Autodesk Inventor part; units mm, degrees
ref_plane "YZ Plane" through (0, 0, 0) normal (1, 0, 0) x (0, 1, 0)
ref_plane "XZ Plane" through (0, 0, 0) normal (0, 1, 0) x (-1, 0, 0)
ref_plane "XY Plane" through (0, 0, 0) normal (0, 0, 1) x (1, 0, 0)
sketch "Sketch1" plane through (0, 0, 0) normal (0, 0, 1) x (1, 0, 0)
  line L0 (0, 0) -> (300, 0)
  line L1 (300, 0) -> (300, 200)
  line L2 (300, 200) -> (0, 200)
  line L3 (0, 200) -> (0, 0)
  dimension "d0" = 300
  dimension "d1" = 200
extrude "Extrusion1" add sketch "Sketch1" along normal blind 12
sketch "Sketch2" plane through (0, 0, 0) normal (0, 0, -1) x (-1, 0, 0)
  line L0 (-250, 150) -> (-50, 150)
  line L1 (-50, 150) -> (-50, 50)
  line L2 (-50, 50) -> (-250, 50)
  line L3 (-250, 50) -> (-250, 150)
  point P0 (0, 0)
  dimension "d4" = 200
  dimension "d5" = 100
extrude "Extrusion2" cut sketch "Sketch2" against normal blind 19
sketch "Sketch3" plane through (0, 0, 12) normal (0, 0, 1) x (1, 0, 0)
  line L0 (0, 0) -> (300, 0)
  line L1 (300, 0) -> (250, 0)
  line L2 (250, 0) -> (250, 200)
  line L3 (250, 200) -> (300, 200)
  line L4 (300, 200) -> (300, 0)
  line L5 (0, 0) -> (50, 0)
  line L6 (50, 0) -> (50, 200)
  line L7 (50, 200) -> (0, 200)
  line L8 (0, 200) -> (0, 0)
  dimension "d8" = 50
  dimension "d9" = 200
  dimension "d10" = 50
  dimension "d11" = 200
extrude "Extrusion3" add sketch "Sketch3" along normal blind 50
sketch "Sketch4" plane through (0, 0, 0) normal (-1, 0, 0) x (0, 0, 1)
  point P0 (0, 0)
sketch "Sketch5" plane through (0, 0, 0) normal (-1, 0, 0) x (0, 0, 1)
  circle A0 centre (37, 35) radius 4
  circle A1 centre (37, 100) radius 6.5
  circle A2 centre (37, 165) radius 4
  point P0 (0, 0)
  dimension "d14" = 8
  dimension "d15" = 13
  dimension "d16" = 8
extrude "Extrusion4" cut sketch "Sketch5" against normal blind 900
chamfer "Chamfer1" distance 5 angle 45 9 edges at (0, 100, 62) (0, 0, 31) (25, 0, 62) (275, 0, 62) (300, 100, 62) (275, 200, 62) (300, 200, 31) (0, 200, 31) (300, 0, 31)
properties part number "base box"
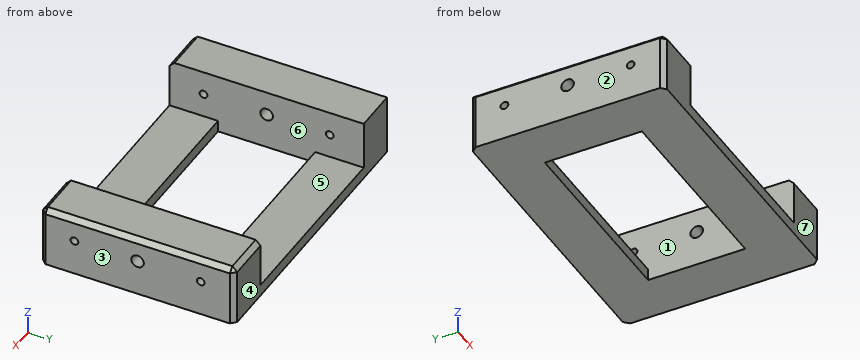
Source: CAD feature listing. Evaluate the final solid. Frame: model axes, mm. Face numbers are marked on the shaded views. A direction names the side the tool comes from. Give positions to 0.01 mm unless a question says otherwise; leave off trailing zeros. Loops run counter-clockwise (first coordinate to the right, second up) from the corner with the lowest first, then second, coordinate; pieces in that order, holes last. Notation, with made-up numbers: (-1, 49) -> (14, 49) arc R16 ccw to (14, 54) -> close; hole circle Ø7 at (-5.5, -1.5). An arc over 180 degrees is marked (long way). Use a Markdown table: item, result. Add a question column.
(1) Ray query, line 1 (Y direction, x = 11, z = 37); line 2 (X direction, y = 96, z = 4); line 3 (Y direction, x = 42, z = 38). Return the intervals inside material, ascending.
(2) First-contact query: pin 1 Ø8 at (x, y) = (200.5, 156.5) entering from +Z. Flat tip, straight axial feed; report the tip coordinate or a pass-through.
(3) Section query D-D (x = 91.5). Output: boundary loops of the cut face in (y, z), then the cut area to 3 significant figures.
(4) Section query A-A (y = 82). Output: boundary loops of the cut face in (x, z).
(5) Pull-direction query (X, two-part tool) for the marked faces 1, 2, 3 and 4; classes: +X half, -X half, draft (parallel to the pull), parting line (faces both ways), or undercut.
(6) Section query C-C (y = 165). Output: boundary loops of the cut face in (x, z).
(7) Access query for the marked faces 5, 6 and 7. Directions: +Z, -Z, +X, -X, +Y, -Y. A direction counts if a zero-diameter tool reaches every point of the face in a straight line with its end or side. Return the directions, or none.
(8) Section query B-B (z = 26). Output: boundary loops of the cut face in (x, y).
Checked values:
| question | item | result |
|---|---|---|
| 1 | line 1 | 0 to 31, 39 to 93.5, 106.5 to 161, 169 to 200 |
| 1 | line 2 | 0 to 50, 250 to 300 |
| 1 | line 3 | 0 to 31.13, 38.87 to 93.58, 106.42 to 161.13, 168.87 to 200 |
| 2 | pin 1 | z = 12 |
| 3 | outline | (0, 0) -> (50, 0) -> (50, 12) -> (0, 12) -> close; (150, 0) -> (200, 0) -> (200, 12) -> (150, 12) -> close |
| 3 | area | 1,200 mm^2 |
| 4 | outline | (0, 0) -> (50, 0) -> (50, 62) -> (5, 62) -> (0, 57) -> close; (250, 0) -> (300, 0) -> (300, 57) -> (295, 62) -> (250, 62) -> close |
| 5 | face 1 | undercut |
| 5 | face 2 | -X half |
| 5 | face 3 | +X half |
| 5 | face 4 | draft |
| 6 | outline | (0, 0) -> (300, 0) -> (300, 33) -> (250, 33) -> (250, 12) -> (50, 12) -> (50, 33) -> (0, 33) -> close; (0, 41) -> (50, 41) -> (50, 62) -> (5, 62) -> (0, 57) -> close; (250, 41) -> (300, 41) -> (300, 57) -> (295, 62) -> (250, 62) -> close |
| 7 | face 5 | +Z, +Y, -Y |
| 7 | face 6 | +Z |
| 7 | face 7 | +Z, -Z, +X, -X, -Y |
| 8 | outline | (0, 5) -> (5, 0) -> (50, 0) -> (50, 200) -> (5, 200) -> (0, 195) -> close; (250, 0) -> (295, 0) -> (300, 5) -> (300, 195) -> (295, 200) -> (250, 200) -> close |
